Work out the finished part from the listing and answer in its coordinate system (mm). Give positions to 0.01 mm unless a question says otherwise; leave off trailing zeros. Loops run counter-clockwise (first coordinate to the right, second up) from the corner with the lowest first, then second, coordinate; pieces in that order, holes last. Notation, with made-up numbers: M -37.75,66.5 L -4.75,66.5 A9 cw -4.75,74.5 Z; hole C 46,64.5 d8. An arc over 180 degrees is marked long. Use a Markdown table: item, result.
```python
from build123d import *

# Parameters (mm, degrees)
CYLINDER071_R               = 1
CYLINDER071_DEPTH           = 16
CYLINDER062_R               = 2
CYLINDER062_DEPTH           = 4
CYLINDER064_R               = 1
CYLINDER064_DEPTH           = 8
CYLINDER069_R               = 1
CYLINDER069_DEPTH           = 67
CYLINDER069_ROLL_ANGLE      = 14.618093
CYLINDER069_PITCH_ANGLE     = -22.769702
CYLINDER069_PLACEMENT_ANGLE = 14.618093
CYLINDER070_R               = 1
CYLINDER070_DEPTH           = 68


with BuildPart() as cylindre067:
    # Cylinder071 → Cylinder071 (new body)
    with BuildSketch(Plane(origin=(-18, 17, -43), x_dir=(1, 0, 0), z_dir=(0, 0, 1))):
        Circle(CYLINDER071_R)
    extrude(amount=CYLINDER071_DEPTH)


with BuildPart() as obj1:
    # Cone002 → Cone002 (revolve)
    with BuildSketch(Plane(origin=(-32, 9, -106), x_dir=(1, 0, 0), z_dir=(0, -1, 0))):
        Polygon((0, 0), (2, 0), (1, 2), (0, 2), align=None)
    revolve(axis=Axis((-32, 9, -106), (0, 0, 1)))


with BuildPart() as fusion035:
    # Cylinder062 → Cylinder062 (new body)
    with BuildSketch(Plane(origin=(-32, 9, -110), x_dir=(1, 0, 0), z_dir=(0, 0, 1))):
        Circle(CYLINDER062_R)
    extrude(amount=CYLINDER062_DEPTH)

    # Fusion029: union obj1
    add(obj1.part)


with BuildPart() as fusion035_1:
    # Fusion029 placement: moved
    add(fusion035.part.moved(Location((14, 8, 62))))

    # Fusion035: union Cylindre067
    add(cylindre067.part)


with BuildPart() as fusion036:
    # Cylinder064 → Cylinder064 (new body)
    with BuildSketch(Plane(origin=(-18, 17, -51), x_dir=(1, 0, 0), z_dir=(0, 0, 1))):
        Circle(CYLINDER064_R)
    extrude(amount=CYLINDER064_DEPTH)

    # Fusion036: union Fusion035
    add(fusion035_1.part)


with BuildPart() as fusion037:
    # Cylinder069 → Cylinder069 (new body)
    with BuildSketch(Plane.XY):
        Circle(CYLINDER069_R)
    extrude(amount=CYLINDER069_DEPTH)


with BuildPart() as fusion037_1:
    # Cylinder069 roll: moved
    add(fusion037.part.rotate(Axis((0, 0, 0), (1, 0, 0)), CYLINDER069_ROLL_ANGLE))


with BuildPart() as fusion037_2:
    # Cylinder069 pitch: moved
    add(fusion037_1.part.rotate(Axis((0, 0, 0), (0, 1, 0)), CYLINDER069_PITCH_ANGLE))


with BuildPart() as fusion037_3:
    # Cylinder069 placement: moved
    add(fusion037_2.part.moved(Location((-18, 17, -27))).rotate(Axis((-18, 17, -27), (0, 0, 1)), CYLINDER069_PLACEMENT_ANGLE))

    # Fusion037: union Fusion036
    add(fusion036.part)


with BuildPart() as fusion038:
    # Cylinder070 → Cylinder070 (new body)
    with BuildSketch(Plane(origin=(-38, -5.6, 32), x_dir=(1, 0, 0), z_dir=(0, 0, 1))):
        Circle(CYLINDER070_R)
    extrude(amount=CYLINDER070_DEPTH)

    # Fusion038: union Fusion037
    add(fusion037_3.part)


solid = fusion038.part
```
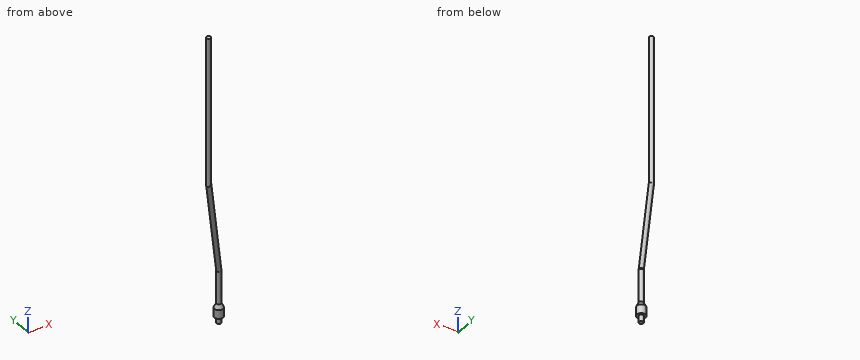
(1) Given P1, Ø12, axis at x = -36, z = 82.5, coming from the +Y side; P2, Ø1.9, axis at x = -38.5, y = -6, coming from the -Z side; P3, Ø2, axis at y = -3, z = 26.5, coming from the -X side, each flat-ended and moving along its own axis, determine where each tip first touches the part or whether it passes through.
Entries:
| item | result |
|---|---|
| P1 | stops at y = -4.6 |
| P2 | stops at z = 29.79 |
| P3 | stops at x = -37.23 |
(2) A cutting plane is placed at A-A (z = 57). Write down the section's boundary in (x, y), and give its area (3 significant figures).
Entries:
| item | result |
|---|---|
| outline | C -38,-5.6 d2 |
| area | 3.14 mm² |
(3) Consider probe 1 along Y at (x, z) = (-25.25, -2.5). Determine where the line is inside the solid, lowest interval first. Write a range as [from, to].
Entries:
| item | result |
|---|---|
| probe 1 | y = [7.35, 8.27] |
